from build123d import *

# Parameters (mm, degrees)
SKETCH_1_W          = 175
SKETCH_1_H          = 70
EXTRUDE_1_DEPTH     = 5
SKETCH_2_R          = 3
SKETCH_2_R_2        = 1.55
CUT_EXTRUDE_1_DEPTH = 10


with BuildPart() as part:
    # 草图1 → 凸台-拉伸1 (new body)
    with BuildSketch(Plane.XY):
        with Locations((87.5, -60)):
            Rectangle(SKETCH_1_W, SKETCH_1_H)
    extrude(amount=EXTRUDE_1_DEPTH)

    # 草图2 → 切除-拉伸1 (cut)
    with BuildSketch(Plane.XY.offset(5)):
        with Locations((87.5, -65.45)):
            Circle(SKETCH_2_R)
        with Locations((69.82233047, -47.77233047)):
            Circle(SKETCH_2_R_2)
        with Locations((105.17766953, -47.77233047)):
            Circle(SKETCH_2_R_2)
        with Locations((105.17766953, -83.12766953)):
            Circle(SKETCH_2_R_2)
        with Locations((69.82233047, -83.12766953)):
            Circle(SKETCH_2_R_2)
    extrude(amount=-CUT_EXTRUDE_1_DEPTH, mode=Mode.SUBTRACT)


solid = part.part
Geometry check sheet. Reference: the model listing, model coordinates, mm. Coordinates: 2 decimals unless noted, no trailing zeros. Write each loop counter-clockwise with the first axis right and the second up, starting at its lowest first coordinate (ties: lowest second). Pieces come first, ordered by that corner, then holes. Notation, with made-up numbers: (18.5, 29) -> (46.5, 29) arc R30 cw to (46.5, 55) -> close; hole circle Ø8 at (64, 25). An arc over 180 degrees is marked (long way). One line per question, with ' | ' between items.
1. Cross-section at A-A on x = 87.5. Record the cut outline in (y, z).
Answers:
outline: (-95, 0) -> (-68.45, 0) -> (-68.45, 5) -> (-95, 5) -> close; (-62.45, 0) -> (-25, 0) -> (-25, 5) -> (-62.45, 5) -> close
2. Cross-section at B-B on y = -65.45. Record the cut outline in (x, z), and give its area (3 significant figures).
Answers:
outline: (0, 0) -> (84.5, 0) -> (84.5, 5) -> (0, 5) -> close; (90.5, 0) -> (175, 0) -> (175, 5) -> (90.5, 5) -> close | area: 845 mm²
3. Thickness scan on probe 1 along Y at (x, z) = (70, 3.75); probe 2 along Y at (x, z) = (87.5, 2); probe 3 along X at (y, z) = (-84.5, 4.35). Record the ranges inside material, lowest first. Write a range as from..to.
Answers:
probe 1: y = -95..-84.67, -81.59..-49.31, -46.23..-25 | probe 2: y = -95..-68.45, -62.45..-25 | probe 3: x = 0..69.1, 70.54..104.46, 105.9..175
4. Depth check by flat-ended pin: pin 1 Ø2.5 at (x, y) = (69.82, -47.77) entering from -Z. Enter the tip coordinate at first touch or a pass-through.
Answers:
pin 1: passes through
5. Draft check along Y on faces 1 (the flat face through (86, -95, 2)), 2 (the cylindrical face through (106.656, -47.307, 2.535)), 3 (the flat face through (86, -25, 2)), 4 (the flat face through (86, -60, 5)). Enter one of: +Y half, -Y half, draft (parallel to the pull), parting line (faces both ways), or undercut.
Answers:
face 1: -Y half | face 2: undercut | face 3: +Y half | face 4: draft
